from build123d import *

# Parameters (mm, degrees)
SKETCH1_W             = 22
SKETCH1_H             = 10
BOSS_EXTRUDE1_DEPTH   = 2.5
F_6_CLEARANCE_HOLE1_D = 3.6576
SKETCH4_W             = 2
SKETCH4_H             = 10
BOSS_EXTRUDE2_DEPTH   = 0.15
FILLET1_R             = 3
CHAMFER1_SIZE         = 0.45


with BuildPart() as part:
    # Sketch1 → Boss-Extrude1 (new body)
    with BuildSketch(Plane(origin=(0, 0, 0), x_dir=(1, 0, 0), z_dir=(0, 1, 0))):
        Rectangle(SKETCH1_W, SKETCH1_H)
    extrude(amount=BOSS_EXTRUDE1_DEPTH)

    # #6 Clearance Hole1 (through all)
    with Locations(Plane(origin=(0, 2.5, 0), x_dir=(1, 0, 0), z_dir=(0, 1, 0))):
        with Locations((7, 0), (-7, 0)):
            Hole(F_6_CLEARANCE_HOLE1_D / 2)

    # Sketch4 → Boss-Extrude2 (add)
    with BuildSketch(Plane.XZ):
        Rectangle(SKETCH4_W, SKETCH4_H)
    extrude(amount=BOSS_EXTRUDE2_DEPTH)

    # Fillet1
    fillet1_edges = [part.edges().sort_by_distance(p)[0] for p in [
        (11, 1.25, 5),
        (-11, 1.25, 5),
        (-11, 1.25, -5),
        (11, 1.25, -5),
    ]]
    fillet(fillet1_edges, radius=FILLET1_R)

    # Chamfer1
    chamfer1_edges = [part.edges().sort_by_distance(p)[0] for p in [
        (4.5, 0, 5),
        (-4.5, 0, -5),
        (11, 0, 0),
        (11, 2.5, 0),
        (4.5, 0, -5),
        (10.121320344, 0, -4.121320344),
        (10.121320344, 0, 4.121320344),
        (-4.5, 0, 5),
        (0, 2.5, 5),
        (0, 2.5, -5),
        (-11, 2.5, 0),
        (-10.121320344, 2.5, 4.121320344),
        (-10.121320344, 2.5, -4.121320344),
        (10.121320344, 2.5, -4.121320344),
        (10.121320344, 2.5, 4.121320344),
        (-11, 0, 0),
        (-10.121320344, 0, 4.121320344),
        (-10.121320344, 0, -4.121320344),
    ]]
    chamfer(chamfer1_edges, length=CHAMFER1_SIZE)


solid = part.part
The listing builds one solid part. Answer for the finished solid, in the listing's coordinates (mm). A direction names the side the tool comes from. Coordinates: 2 decimals unless noted, no trailing zeros. Loops run counter-clockwise (first coordinate to the right, second up) from the corner with the lowest first, then second, coordinate; pieces in that order, holes last.
1) A tool of negligible diameter and unlimited length cuts with its end or side. For faces 1 (the face through (5, 0, 0)), 2 (the face through (-11, 1, 0)), from which of +Z, -Z, +X, -X, +Y, -Y can it reach the whole face along a straight path? Write none if from no direction.
2) Find section B-B on y = 1.75. Write down the section's boundary in (x, z), then the cut area to 3 significant figures.
3) Find section D-D on x = 1.25. Write down the section's boundary in (y, z).
4) Find section C-C on z = 0. Write down the section's boundary in (x, y), then the cut area to 3 significant figures.
5) Find the intervals of material crossed by L1, parallel to Z at x = 7, y = 0.5; L2, parallel to X at y = 1.5, z = 1; L3, parallel to X at y = 1.1, z = -1.25, in increasing order.
6) Flat-ended cylindrical pins translate along their axes: pin 1 Ø0.7 at (y, z) = (0, 1.5) entering from +X; pin 2 Ø3 at (x, z) = (-7, 0) entering from -Y. Find the tip coordinate at first contact, or state that the pin passes through.
7) Determine the mould class of faces 3 (the face through (-5.549, 1.232, 1.113)), 4 (the face through (-5, 0, 0)), 5 (the face through (-10.14, 1.26, -4.1)), 6 (the face through (-9.873, 0.128, 3.914)) for opening direction Z: pulls with the +Z half, pulls with the -Z half, needs draft (parallel to the pull), parting line crosses it, or undercut.
8) Find section A-A on x = -7. Write down the section's boundary in (y, z).
Values:
1. face 1: +Z, -Z, +X, -Y
1. face 2: +Z, -Z, -X, +Y, -Y
2. outline: (-11, -2) arc R3 ccw to (-8, -5) - (8, -5) arc R3 ccw to (11, -2) - (11, 2) arc R3 ccw to (8, 5) - (-8, 5) arc R3 ccw to (-11, 2) - close; hole circle Ø3.66 at (-7, 0); hole circle Ø3.66 at (7, 0)
2. area: 191 mm2
3. outline: (0, -4.55) - (0.45, -5) - (2.05, -5) - (2.5, -4.55) - (2.5, 4.55) - (2.05, 5) - (0.45, 5) - (0, 4.55) - close
4. outline: (-11, 0.45) - (-10.55, 0) - (-8.83, 0) - (-8.83, 2.5) - (-10.55, 2.5) - (-11, 2.05) - close; (-5.17, 0) - (-1, 0) - (-1, -0.15) - (1, -0.15) - (1, 0) - (5.17, 0) - (5.17, 2.5) - (-5.17, 2.5) - close; (8.83, 0) - (10.55, 0) - (11, 0.45) - (11, 2.05) - (10.55, 2.5) - (8.83, 2.5) - close
4. area: 36.6 mm2
5. L1: z = -5 to -1.83, 1.83 to 5
5. L2: x = -11 to -8.53, -5.47 to 5.47, 8.53 to 11
5. L3: x = -11 to -8.33, -5.67 to 5.67, 8.33 to 11
6. pin 1: stops at x = 10.9
6. pin 2: passes through
7. face 3: undercut
7. face 4: needs draft
7. face 5: pulls with the -Z half
7. face 6: pulls with the +Z half
8. outline: (0, -4.55) - (0.45, -5) - (2.05, -5) - (2.5, -4.55) - (2.5, -1.83) - (0, -1.83) - close; (0, 1.83) - (2.5, 1.83) - (2.5, 4.55) - (2.05, 5) - (0.45, 5) - (0, 4.55) - close
